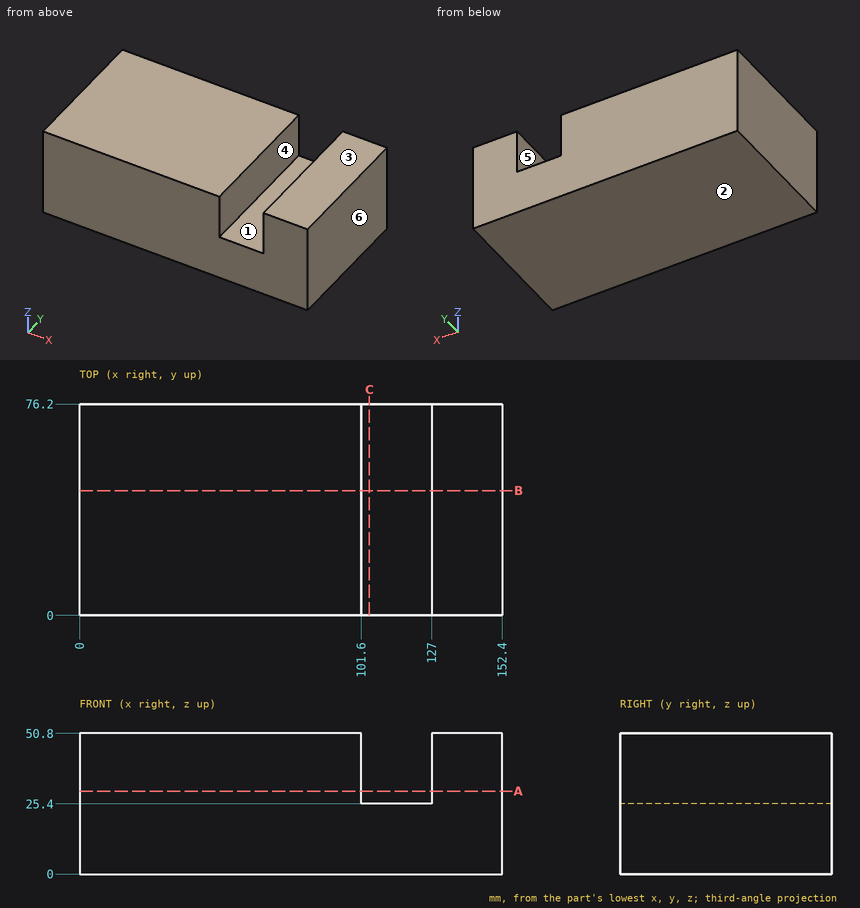
Geometry check sheet. Reference: drawing and pictorial views, mm from the part's lowest x, y, z. A direction names the side the tool comes from. Give positions to 0.01 mm unless a question says otherwise; leave off trailing zeros. Write each loop counter-clockwise with the first axis right and the second up, starting at its lowest first coordinate (ties: lowest second). Pieces come first, ordered by that corner, then holes. Notation, with made-up numbers: (2, 46.5) - (36, 46.5) arc R27 cw to (36, 71.5) - close; hole circle Ø4 at (49, 6). An arc over 180 degrees is marked (long way). Use a Markdown table: item, result.
Q1. Section check A-A, the plane z = 30. Enter the section's corners in (x, y), then the cut area to 3 significant figures.
Computed:
| item | result |
|---|---|
| outline | (0, 0) - (101.6, 0) - (101.6, 76.2) - (0, 76.2) - close; (127, 0) - (152.4, 0) - (152.4, 76.2) - (127, 76.2) - close |
| area | 9,680 mm² |
Q2. Set-up check for the marked faces 1 and 2: record each of +Z, -Z, +X, -X, +Y, -Y from which the full face is reachable in a straight line by a thin tool's end or side.
Computed:
| item | result |
|---|---|
| face 1 | +Z, +Y, -Y |
| face 2 | -Z, +X, -X, +Y, -Y |
Q3. Section check B-B, the plane y = 45. Enter the section's corners in (x, z).
Computed:
| item | result |
|---|---|
| outline | (0, 0) - (152.4, 0) - (152.4, 50.8) - (127, 50.8) - (127, 25.4) - (101.6, 25.4) - (101.6, 50.8) - (0, 50.8) - close |
Q4. Section check C-C, the plane x = 104.5. Enter the section's corners in (y, z).
Computed:
| item | result |
|---|---|
| outline | (0, 0) - (76.2, 0) - (76.2, 25.4) - (0, 25.4) - close |
Q5. Thickness scan on L1, parallel to X at y = 12, z = 46; L2, parallel to Z at x = 123.5, y = 53. Record the ranges inside material, lowest first. Write a range as [from, to].
Computed:
| item | result |
|---|---|
| L1 | x = [0, 101.6], [127, 152.4] |
| L2 | z = [0, 25.4] |
Q6. Draft check along X on the marked faces 3, 4, 5 and 6. Enter one of: pulls with the +X half, pulls with the -X half, needs draft (parallel to the pull), parting line crosses it, or undercut.
Computed:
| item | result |
|---|---|
| face 3 | needs draft |
| face 4 | undercut |
| face 5 | undercut |
| face 6 | pulls with the +X half |
